Part model, mm, in its own coordinate system. A direction names the side the tool comes from. Give positions to 0.01 mm unless a question says otherwise; leave off trailing zeros. Loops run counter-clockwise (first coordinate to the right, second up) from the corner with the lowest first, then second, coordinate; pieces in that order, holes last. Notation, with made-up numbers: (65.5, 5) -> (79.5, 5) arc R20 ccw to (79.5, 9) -> close; hole circle Ø10 at (28.25, 38.25). An arc over 180 degrees is marked (long way). One line per question, with ' | ' between items.
```python
from build123d import *

# Parameters (mm, degrees)
BOSS_EXTRUDE1_DEPTH              = 254
FILLET1_R                        = 1.27
FILLET2_R                        = 4.445
F_17_64_0_26563_DIAMETER_HOLE1_D = 6.747002
FILLET3_R                        = 6.35


with BuildPart() as part:
    # Sketch1 → Boss-Extrude1 (new body)
    with BuildSketch(Plane(origin=(0, 0, 0), x_dir=(0, 0, -1), z_dir=(1, 0, 0))):
        Polygon((0, 0), (28.575, 0), (28.575, -11.43), (53.975, -11.43), (53.975, -14.605), (25.4, -14.605), (25.4, -3.175), (0, -3.175), align=None)
    extrude(amount=BOSS_EXTRUDE1_DEPTH)

    # Fillet1
    fillet1_edges = [part.edges().sort_by_distance(p)[0] for p in [
        (127, -11.43, -28.575),
        (127, -3.175, -25.4),
    ]]
    fillet(fillet1_edges, radius=FILLET1_R)

    # Fillet2
    fillet2_edges = [part.edges().sort_by_distance(p)[0] for p in [
        (127, 0, -28.575),
        (127, -14.605, -25.4),
    ]]
    fillet(fillet2_edges, radius=FILLET2_R)

    # 17/64 (0.26563) Diameter Hole1 (through all)
    with Locations(Plane(origin=(0, 0, 0), x_dir=(1, 0, 0), z_dir=(0, 1, 0))):
        with Locations((241.3, 9.525), (12.7, 9.525)):
            Hole(F_17_64_0_26563_DIAMETER_HOLE1_D / 2)

    # Fillet3
    fillet3_edges = [part.edges().sort_by_distance(p)[0] for p in [
        (0, -1.5875, 0),
        (254, -13.0175, -53.975),
        (254, -1.5875, 0),
        (0, -13.0175, -53.975),
    ]]
    fillet(fillet3_edges, radius=FILLET3_R)


solid = part.part
```
1) Saw through at B-B (x = 173). Give the cut face in (y, z) (3 decimals), and give its area (3 significant figures).
Found:
outline: (-14.605, -53.975) -> (-11.43, -53.975) -> (-11.43, -29.845) arc R1.27 cw to (-10.16, -28.575) -> (-4.445, -28.575) arc R4.445 ccw to (0, -24.13) -> (0, 0) -> (-3.175, 0) -> (-3.175, -24.13) arc R1.27 cw to (-4.445, -25.4) -> (-10.16, -25.4) arc R4.445 ccw to (-14.605, -29.845) -> close | area: 200 mm2
2) Drill centre lines: line 1 (Z direction, x = 117.5, y = -5.25) (3 decimals); line 2 (Y direction, x = 71.5, z = -30.5) (3 decimals); line 3 (Y direction, x = 32.5, z = -20) (3 decimals). Where is each one in solid material? Low to high.
Found:
line 1: -28.575 to -25.4 | line 2: -14.605 to -11.43 | line 3: -3.175 to 0
3) Saw through at A-A (x = 12.7). Give the cut face in (y, z) (1 decimal), and give its area (3 significant figures).
Found:
outline: (-14.6, -54) -> (-11.4, -54) -> (-11.4, -29.8) arc R1.3 cw to (-10.2, -28.6) -> (-4.4, -28.6) arc R4.4 ccw to (0, -24.1) -> (0, -12.9) -> (-3.2, -12.9) -> (-3.2, -24.1) arc R1.3 cw to (-4.4, -25.4) -> (-10.2, -25.4) arc R4.4 ccw to (-14.6, -29.8) -> close; (-3.2, -6.2) -> (0, -6.2) -> (0, 0) -> (-3.2, 0) -> close | area: 178 mm2
4) Pull direction X, two halves, no side cores. Call faces 1 (the flat face through (125, -14.605, -42)), 2 (the cylindrical face through (1.811, -13.04, -52.065)), 3 (the cylindrical face through (9.584, -1.61, -8.233)): pulls with the +X half, pulls with the -X half, needs draft (parallel to the pull), parting line crosses it, or undercut.
Found:
face 1: needs draft | face 2: pulls with the -X half | face 3: undercut
5) Pin check, flat tips, straight feed: P1, Ø1.7, axis at x = 79.5, y = -8, coming from the +Z side; P2, Ø8, axis at x = 241.3, z = -9.525, coming from the -Y side (3 decimals); P3, Ø4, axis at x = 150.5, z = -44, coming from the +Y side; P4, Ø5, axis at y = -5, z = -25.5, coming from the -X side. Stop position of each tip, or through.
Found:
P1: z = -25.4 | P2: y = -3.175 | P3: y = -11.43 | P4: x = 0
6) Tool access for faces 4 (the flat face through (125, -7, -28.575)), 5 (the cylindrical face through (252.189, -13.04, -52.065)), 6 (the flat face through (125, -3.175, -12)): list every direction of +Z, -Z, +X, -X, +Y, -Y with a clear straight run to the whole face (end or side of a thin tool).
Found:
face 4: -Z, +X, -X, +Y | face 5: -Z, +X, +Y, -Y | face 6: +Z, +X, -X, -Y
7) Saw through at C-C (z = -16.5). Give the cut face in (x, y) (3 decimals), and give its area (3 significant figures).
Found:
outline: (0, -3.175) -> (254, -3.175) -> (254, 0) -> (0, 0) -> close | area: 806 mm2
